For this review, take the finished solid that the model builds, in its own axes (mm). Face numbers are marked on the shaded views. A direction names the side the tool comes from. Round coordinates to 2 decimals unless told otherwise and drop trailing zeros. Write each loop counter-clockwise with the first axis right and the second up, starting at its lowest first coordinate (ties: lowest second). Pieces come first, ordered by that corner, then holes. Notation, with made-up numbers: M 34.5,39 L 40.5,39 A15 cw 40.5,64 Z; hole C -21,-18.75 d10. An arc over 180 degrees is marked long. Answer in a Markdown table with one row per item.
```python
from build123d import *

# Parameters (mm, degrees)
SKETCH1_W                    = 449.326
SKETCH1_H                    = 127
BASE_FLANGE1_DEPTH           = 3.175
EDGE_FLANGE1_STRIP_W         = 14.1732
EDGE_FLANGE1_STRIP_H         = 3.175
EDGE_FLANGE1_STRIP_CUT_DEPTH = 449.326
EDGE_FLANGE1_DEPTH           = 449.326
CUT_EXTRUDE1_DEPTH           = 484.892399482
SKETCH10_W                   = 25.4
SKETCH10_H                   = 3.175
BOSS_EXTRUDE1_DEPTH          = 25.4
F_1_4_CLEARANCE_HOLE1_D      = 6.7564
F_1_4_CLEARANCE_HOLE1_DEPTH  = 25.4
F_1_4_CLEARANCE_HOLE1_TIP    = 2.029827343


# Sheet-metal steps are written as plain solids
with BuildPart() as part:
    # Sketch1 → Base-Flange1 (new body)
    with BuildSketch(Plane(origin=(0, 0, 0), x_dir=(1, 0, 0), z_dir=(0, 1, 0))):
        with Locations((224.663, 63.5)):
            Rectangle(SKETCH1_W, SKETCH1_H)
    extrude(amount=-BASE_FLANGE1_DEPTH)

    # Edge-Flange1 strip (across the edge) → Edge-Flange1 strip cut (cut)
    with BuildSketch(Plane(origin=(449.326, 0, -127), x_dir=(0, 0, 1), z_dir=(-1, 0, 0))):
        with Locations((-3.175, -1.5875)):
            Rectangle(EDGE_FLANGE1_STRIP_W, EDGE_FLANGE1_STRIP_H)
    extrude(amount=EDGE_FLANGE1_STRIP_CUT_DEPTH, mode=Mode.SUBTRACT)

    # Edge-Flange1 section (across the edge) → Edge-Flange1 (add)
    with BuildSketch(Plane(origin=(449.326, 0, -127), x_dir=(0, 0, 1), z_dir=(-1, 0, 0))):
        with BuildLine():
            Line((0, 0.7366), (0, 127))
            Line((0, 127), (3.175, 127))
            Line((3.175, 127), (3.175, 0.7366))
            ThreePointArc((3.175, 0.7366), (3.390745145, 0.215745145), (3.9116, 0))
            Line((3.9116, 0), (3.9116, -3.175))
            ThreePointArc((3.9116, -3.175), (1.145681115, -2.029318885), (0, 0.7366))
        make_face()
    extrude(amount=EDGE_FLANGE1_DEPTH)

    # Sketch9 → Cut-Extrude1 (cut, through all)
    with BuildSketch(Plane(origin=(0, 0, -127), x_dir=(-1, 0, 0), z_dir=(0, 0, -1))):
        with BuildLine():
            Line((-433.324, 107.95), (-433.324, 127))
            Line((-433.324, 127), (-439.928, 127))
            Line((-439.928, 127), (-439.928, 107.95))
            ThreePointArc((-439.928, 107.95), (-436.626, 104.648), (-433.324, 107.95))
        make_face()
        with BuildLine():
            Line((-16.002, 107.95), (-16.002, 127))
            Line((-16.002, 127), (-9.398, 127))
            Line((-9.398, 127), (-9.398, 107.95))
            ThreePointArc((-9.398, 107.95), (-12.7, 104.648), (-16.002, 107.95))
        make_face()
    extrude(amount=-CUT_EXTRUDE1_DEPTH, mode=Mode.SUBTRACT)

    # Sketch10 → Boss-Extrude1 (add)
    with BuildSketch(Plane.XY):
        with Locations((436.626, -1.5875)):
            Rectangle(SKETCH10_W, SKETCH10_H)
        with Locations((12.7, -1.5875)):
            Rectangle(SKETCH10_W, SKETCH10_H)
    extrude(amount=BOSS_EXTRUDE1_DEPTH)

    # 1/4 Clearance Hole1
    with Locations(Plane(origin=(12.7, -3.175, 12.7), x_dir=(0, 0, -1), z_dir=(0, -1, 0))):
        with Locations((0, 0), (0, 423.926)):
            Hole(F_1_4_CLEARANCE_HOLE1_D / 2, depth=F_1_4_CLEARANCE_HOLE1_DEPTH)
            with Locations((0, 0, -(F_1_4_CLEARANCE_HOLE1_DEPTH + F_1_4_CLEARANCE_HOLE1_TIP / 2))):  # 118° drill point
                Cone(0, F_1_4_CLEARANCE_HOLE1_D / 2, F_1_4_CLEARANCE_HOLE1_TIP, mode=Mode.SUBTRACT)


solid = part.part
```
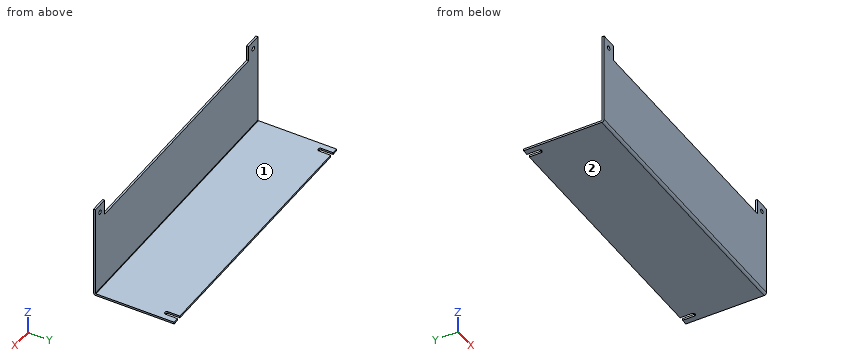
Q1. For probe 1 along X at (y, z) = (-1.25, 12.7); probe 2 along X at (y, z) = (-2, 12); probe 3 along Y at (x, z) = (104.5, -4.5) (3 decimals), list the stretches that pass through material, from the lowest coordinate up.
Found:
| item | result |
|---|---|
| probe 1 | 0 to 9.32, 16.08 to 25.4, 423.93 to 433.25, 440 to 449.33 |
| probe 2 | 0 to 9.4, 16 to 25.4, 423.93 to 433.32, 439.93 to 449.33 |
| probe 3 | -3.175 to 0 |
Q2. Take a section at A-A (x = 166.5). State the section outline as (y, z) points (3 decimals), then the cut area to 3 significant figures.
Found:
| item | result |
|---|---|
| outline | M -3.175,-123.088 A3.912 ccw 0.737,-127 L 127,-127 L 127,-123.825 L 0.737,-123.825 A0.737 cw 0,-123.088 L 0,0 L -3.175,0 Z |
| area | 803 mm² |
Q3. Take a section at B-B (z = -30.5). State the section outline as (x, y) points (3 decimals).
Found:
| item | result |
|---|---|
| outline | M 0,-3.175 L 449.326,-3.175 L 449.326,0 L 0,0 Z |
Q4. Machinability: for the marked faces 1 and 2, which of the approach directions +Z, -Z, +X, -X, +Y, -Y give a long, thin tool a straight path to every point of the face, cutting with its end or side? Answer none if there is none.
Found:
| item | result |
|---|---|
| face 1 | +Z, +X, -X, +Y |
| face 2 | -Z, +X, -X, +Y, -Y |
Q5. Take a section at C-C (y = 97). State the section outline as (x, z) points (3 decimals), then the cut area to 3 significant figures.
Found:
| item | result |
|---|---|
| outline | M 0,-127 L 449.326,-127 L 449.326,-123.825 L 0,-123.825 Z |
| area | 1,430 mm² |
Q6. Insertion check: P1, Ø4, axis at x = 317.5, y = 80, coming from the +Z side (3 decimals); P2, Ø6, axis at x = 12.7, z = 12.7, coming from the -Y side; P3, Ø8, axis at x = 354, z = -108, coming from the +Y side; P4, Ø3.5, axis at x = 249, y = -2, coming from the +Z side. Each pin has a flat end and moves straight along its axis. Give the tip position at first contact, or say it passes through.
Found:
| item | result |
|---|---|
| P1 | z = -123.825 |
| P2 | through |
| P3 | y = 0 |
| P4 | z = 0 |
